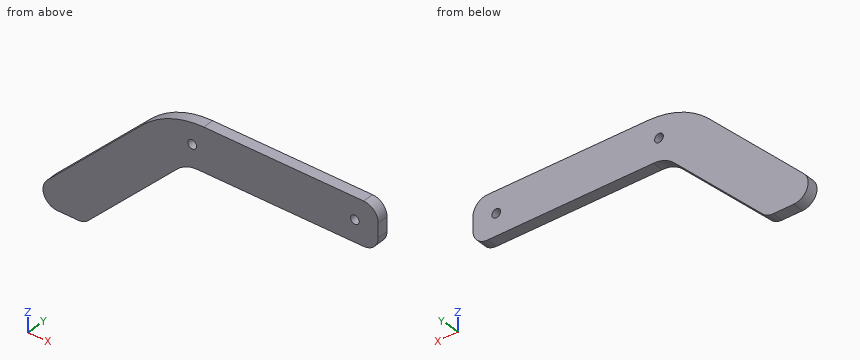
from build123d import *

# Parameters (mm, degrees)
F0_R     = 7.5
F1_DEPTH = 19.05


with BuildPart() as f1:
    # F0 (on Front) → F1 (new body)
    with BuildSketch(Plane.XZ):
        with BuildLine():
            ThreePointArc((-25, 0), (-7.32233, 7.32233), (0, 25))
            Line((0, 25), (0, 50))
            ThreePointArc((0, 50), (-7.32233, 67.67767), (-25, 75))
            Line((-25, 75), (-300, 75))
            ThreePointArc((-300, 75), (-357.402515, 63.58193), (-406.066017, 31.066017))
            Line((-406.066017, 31.066017), (-569.454365, -132.32233))
            ThreePointArc((-569.454365, -132.32233), (-574.873684, -159.567086), (-551.776695, -175))
            Line((-551.776695, -175), (-516.421356, -175))
            ThreePointArc((-516.421356, -175), (-506.85427, -173.096988), (-498.743687, -167.67767))
            Line((-498.743687, -167.67767), (-345.710678, -14.644661))
            ThreePointArc((-345.710678, -14.644661), (-329.489511, -3.806023), (-310.355339, 0))
            Line((-310.355339, 0), (-25, 0))
        make_face()
        with Locations((-320, 37.5)):
            Circle(F0_R, mode=Mode.SUBTRACT)
        with Locations((-40, 37.5)):
            Circle(F0_R, mode=Mode.SUBTRACT)
    extrude(amount=F1_DEPTH)


solid = f1.part
The listing builds one solid part. Answer for the finished solid, in the listing's coordinates (mm). Coordinates: 2 decimals unless noted, no trailing zeros. Order: outer loops, then holes, each group sorted by start corner. A loop starts at its lowest first (then second) coordinate and runs counter-clockwise, first axis right, second up.
Q1. A cutting plane is placed at A-A, the plane x = -40. Write down the section's boundary in (y, z).
Q2. A cutting plane is placed at C-C, the plane z = 37.5. Write down the section's boundary in (x, y), and give its area (3 significant figures).
Q3. Given P1, Ø2, axis at x = -313, y = -9, coming from the -Z side; P2, Ø6, axis at x = -309.5, y = -16, coming from the +Z side; P3, Ø8, axis at y = -7.5, z = -123.5, coming from the -X side; P4, Ø9, axis at x = -320, z = 37.5, coming from the +Y side, each flat-ended and moving along its own axis, determine where each tip first touches the part or whether it passes through.
Q4. Consider line 1 (Z direction, x = -40, y = -4); line 2 (Z direction, x = -94, y = -13.25); line 3 (Z direction, x = -320, y = -13.5). Determine where each line is inside the solid, lowest interval first.
Q5. A cutting plane is placed at B-B, the plane y = -9.25. Write down the section's boundary in (x, z).
Q6. A cutting plane is placed at D-D, the plane z = -38. Write down the section's boundary in (x, y).
Answers follow:
1. outline: (-19.05, 0) - (0, 0) - (0, 30) - (-19.05, 30) - close; (-19.05, 45) - (0, 45) - (0, 75) - (-19.05, 75) - close
2. outline: (-399.22, -19.05) - (-327.5, -19.05) - (-327.5, 0) - (-399.22, 0) - close; (-312.5, -19.05) - (-47.5, -19.05) - (-47.5, 0) - (-312.5, 0) - close; (-32.5, -19.05) - (0, -19.05) - (0, 0) - (-32.5, 0) - close
2. area: 7,030 mm2
3. P1: stops at z = -0.13
3. P2: stops at z = 74.86
3. P3: stops at x = -564.63
3. P4: passes through
4. line 1: z = 0 to 30, 45 to 75
4. line 2: z = 0 to 75
4. line 3: z = -0.94 to 30, 45 to 73.66
5. outline: (-569.45, -132.32) arc R25 ccw to (-551.78, -175) - (-516.42, -175) arc R25 ccw to (-498.74, -167.68) - (-345.71, -14.64) arc R50 cw to (-310.36, 0) - (-25, 0) arc R25 ccw to (0, 25) - (0, 50) arc R25 ccw to (-25, 75) - (-300, 75) arc R150 ccw to (-406.07, 31.07) - close; hole circle Ø15 at (-320, 37.5); hole circle Ø15 at (-40, 37.5)
6. outline: (-475.13, -19.05) - (-369.07, -19.05) - (-369.07, 0) - (-475.13, 0) - close
